The listing builds one solid part. Answer for the finished solid, in the listing's coordinates (mm). A direction names the side the tool comes from. Round coordinates to 2 decimals unless told otherwise and drop trailing zeros. Loops run counter-clockwise (first coordinate to the right, second up) from the corner with the lowest first, then second, coordinate; pieces in that order, holes last. Notation, with made-up numbers: (-40, -8.75) - (13, -8.75) arc R10 ccw to (13, 4.25) - close; hole circle Ø8 at (-30, 15). An arc over 180 degrees is marked (long way). Write item = value, one per line. Start each with the question number.
1) Section A-A, the plane x = -25.4 is taken. Determine the outline of the cut face in (y, z).
2) Section B-B, the plane y = -17.78 is taken. Give the number of separate pieces and of enclosed holes in the cut face, and give its area (3 significant figures).
3) For a pull along Z with two mould halves and no side action, classify faces 1 (the cylindrical face through (35.562, -17.668, 3.863)), 2 (the cylindrical face through (42.38, -8.557, 4.117)), 3 (the flat face through (-7, 5.08, 6)), 4 (the flat face through (1, 0, 12.032)) as released by +Z, released by -Z, zero draft, split by the parting line, or undercut.
4) Given pin 1 Ø4 at (x, y) = (-13, -18.5) entering from +Z; pin 2 Ø1.7 at (y, z) = (-0.5, 7.5) entering from -X (3 decimals); pin 3 Ø1.6 at (x, y) = (8.5, 5.5) entering from -Z, each flat-ended and moving along its own axis, determine where each tip first touches the part or whether it passes through.
5) A tool of negligible diameter and unlimited length cuts with its end or side. For faces 5 (the flat face through (-1, 25.4, 4)), 6 (the flat face through (43, 5.08, 6)), from which of +Z, -Z, +X, -X, +Y, -Y can it reach the whole face along a straight path? Write none if from no direction.
6) Section C-C, the plane z = 8.75 is taken. Determine the outline of the cut face in (x, y) (3 decimals), and give its area (3 significant figures).
7) Section D-D, the plane y = 13 is taken. Determine the outline of the cut face in (x, z) (3 decimals).
8) Straight lines are drawn through the part: line 1 along Y through (x, z) = (0, 2.25); line 2 along Y through (x, z) = (-38.1, 6); line 3 along Z through (x, y) = (35.5, -1). For each, find the intervals that lie inside material, in ascending order.
from build123d import *

# Parameters (mm, degrees)
F0_W      = 95.25
F0_H      = 50.8
F1_DEPTH  = 7.62
F2_R      = 2.54
F3_DEPTH  = 7.621
F4_W      = 10.16
F4_H      = 5.08
F5_DEPTH  = 95.251
F8_R      = 1.27
F9_DEPTH  = 27.2604090512
F12_R     = 1.27
F13_DEPTH = 29.4601135768
F15_DEPTH = 95.25
F16_W     = 2.54
F16_H     = 10.16


with BuildPart() as f1:
    # F0 (on Top) → F1 (new body)
    with BuildSketch(Plane.XY):
        Rectangle(F0_W, F0_H)
    extrude(amount=F1_DEPTH)

    # F2 (on face) → F3 (cut, through all)
    with BuildSketch(Plane.XY.offset(7.62)):
        with Locations((-38.1, 17.78)):
            Circle(F2_R)
        with Locations((-38.1, -17.78)):
            Circle(F2_R)
        with Locations((-25.4, 17.78)):
            Circle(F2_R)
        with Locations((-25.4, -17.78)):
            Circle(F2_R)
        with Locations((-12.7, 17.78)):
            Circle(F2_R)
        with Locations((-12.7, -17.78)):
            Circle(F2_R)
        with Locations((0, 17.78)):
            Circle(F2_R)
        with Locations((0, -17.78)):
            Circle(F2_R)
        with Locations((12.7, 17.78)):
            Circle(F2_R)
        with Locations((12.7, -17.78)):
            Circle(F2_R)
        with Locations((25.4, 17.78)):
            Circle(F2_R)
        with Locations((25.4, -17.78)):
            Circle(F2_R)
        with Locations((38.1, 17.78)):
            Circle(F2_R)
        with Locations((38.1, -17.78)):
            Circle(F2_R)
    extrude(amount=-F3_DEPTH, mode=Mode.SUBTRACT)

    # F4 (on face) → F5 (cut, through all)
    with BuildSketch(Plane.YZ.offset(47.625)):
        with Locations((0, 7.62)):
            Rectangle(F4_W, F4_H)
    extrude(amount=-F5_DEPTH, mode=Mode.SUBTRACT)

    # F8 (on face) → F9 (cut, through all)
    with BuildSketch(Plane(origin=(0, -7.2797045256, 12.6088181024), x_dir=(1, 0, 0), z_dir=(0, 0.5, -0.8660254038))):
        with Locations((-42.545, -8.2094090512)):
            Circle(F8_R)
        with Locations((-32.385, -8.2094090512)):
            Circle(F8_R)
        with Locations((-22.225, -8.2094090512)):
            Circle(F8_R)
        with Locations((-12.065, -8.2094090512)):
            Circle(F8_R)
        with Locations((-1.905, -8.2094090512)):
            Circle(F8_R)
        with Locations((8.255, -8.2094090512)):
            Circle(F8_R)
        with Locations((18.415, -8.2094090512)):
            Circle(F8_R)
        with Locations((28.575, -8.2094090512)):
            Circle(F8_R)
        with Locations((38.735, -8.2094090512)):
            Circle(F8_R)
        with Locations((48.895, -8.2094090512)):
            Circle(F8_R)
    extrude(amount=F9_DEPTH, mode=Mode.SUBTRACT)

    # F12 (on face) → F13 (cut, through all)
    with BuildSketch(Plane(origin=(0, 8.3795567884, 14.5138181024), x_dir=(1, 0, 0), z_dir=(0, -0.5, -0.8660254038))):
        with Locations((42.545, 8.2094090512)):
            Circle(F12_R)
        with Locations((32.385, 8.2094090512)):
            Circle(F12_R)
        with Locations((22.225, 8.2094090512)):
            Circle(F12_R)
        with Locations((12.065, 8.2094090512)):
            Circle(F12_R)
        with Locations((1.905, 8.2094090512)):
            Circle(F12_R)
        with Locations((-8.255, 8.2094090512)):
            Circle(F12_R)
        with Locations((-18.415, 8.2094090512)):
            Circle(F12_R)
        with Locations((-28.575, 8.2094090512)):
            Circle(F12_R)
        with Locations((-38.735, 8.2094090512)):
            Circle(F12_R)
        with Locations((-48.895, 8.2094090512)):
            Circle(F12_R)
    extrude(amount=F13_DEPTH, mode=Mode.SUBTRACT)

    # F14 (on face) → F15 (join, through all)
    with BuildSketch(Plane.YZ.offset(47.625)):
        Polygon((-7.62, 12.0324302436), (-7.62, 7.62), (-5.08, 7.62), (0, 10.7624302436), (5.08, 7.62), (7.62, 7.62), (7.62, 12.0324302436), align=None)
    extrude(amount=-F15_DEPTH)

    # F16 (on face) → F17 (join, up to the next surface of F1)
    with BuildSketch(Plane.XY.offset(5.08)):
        with Locations((46.355, 0)):
            Rectangle(F16_W, F16_H)
    extrude(until=Until.NEXT)


solid = f1.part
Geometry check:
q1.outline = (-25.4, 0) - (-20.32, 0) - (-20.32, 7.62) - (-25.4, 7.62) - close; (-15.24, 0) - (15.24, 0) - (15.24, 7.62) - (7.62, 7.62) - (7.62, 12.03) - (-7.62, 12.03) - (-7.62, 7.62) - (-15.24, 7.62) - close; (20.32, 0) - (25.4, 0) - (25.4, 7.62) - (20.32, 7.62) - close; hole (-5.08, 5.08) - (5.08, 5.08) - (5.08, 7.62) - (0, 10.76) - (-5.08, 7.62) - close
q2.separate_pieces = 8
q2.enclosed_holes = 0
q2.area = 455 mm2
q3.face_1 = zero draft
q3.face_2 = undercut
q3.face_3 = undercut
q3.face_4 = released by +Z
q4.pin_1 = 7.62
q4.pin_2 = 45.085
q4.pin_3 = 0
q5.face_5 = +Z, -Z, +X, -X, +Y
q5.face_6 = -X
q6.outline = (-47.625, -7.62) - (47.625, -7.62) - (47.625, 7.62) - (-47.625, 7.62) - (-47.625, 3.253) - (45.085, 3.253) - (45.085, -3.253) - (-47.625, -3.253) - close
q6.area = 848 mm2
q7.outline = (-47.625, 0) - (47.625, 0) - (47.625, 7.62) - (-47.625, 7.62) - close
q8.line_1 = -25.4 to -20.32, -15.24 to 15.24, 20.32 to 25.4
q8.line_2 = -25.4 to -20.32, -15.24 to -7.29, 5.08 to 15.24, 20.32 to 25.4
q8.line_3 = 0 to 5.08, 10.14 to 12.03
